Work out the finished part from the listing and answer in its coordinate system (mm). Round coordinates to 2 decimals unless told otherwise and drop trailing zeros. Order: outer loops, then holes, each group sorted by start corner. A loop starts at its lowest first (then second) coordinate and runs counter-clockwise, first axis right, second up. Notation, with made-up numbers: M -29.5,-27 L -21.5,-27 A11 cw -21.5,-23 Z; hole C 8.5,-34.75 d9. An arc over 180 degrees is marked long. Answer as a JSON object with one key per item and string values. Group by question number.
from build123d import *

# Parameters (mm, degrees)
F0_R      = 43.786601
F1_DEPTH  = 63.5
F2_R      = 36.948177
F3_DEPTH  = 127.001
F4_R      = 14.964631
F5_DEPTH  = 177.8
F6_R      = 10.234569
F7_DEPTH  = 177.8
F8_DEPTH  = 127.001
F10_DEPTH = 21.80281
F11_R     = 13.282854
F11_R_2   = 9.414952
F12_DEPTH = 119.06572
F13_R     = 8.242853
F14_DEPTH = 126.54868
F15_R     = 37.892403
F16_DEPTH = 63.501
F17_R     = 10.259839
F18_DEPTH = 185.08291
F19_DEPTH = 161.75664


with BuildPart() as f1:
    # F0 (on Front) → F1 (new body, symmetric)
    with BuildSketch(Plane.XZ):
        Circle(F0_R)
    extrude(amount=F1_DEPTH, both=True)

    # F2 (on face) → F3 (cut, through all)
    with BuildSketch(Plane.XZ.offset(63.5)):
        Circle(F2_R)
    extrude(amount=-F3_DEPTH, mode=Mode.SUBTRACT)

    # F4 (on Right) → F5 (join)
    with BuildSketch(Plane.YZ):
        with Locations((43.817297, 0)):
            Circle(F4_R)
    extrude(amount=F5_DEPTH)

    # F6 (on face) → F7 (cut)
    with BuildSketch(Plane.YZ.offset(177.8)):
        with Locations((43.817297, 0)):
            Circle(F6_R)
    extrude(amount=-F7_DEPTH, mode=Mode.SUBTRACT)

    # F2 (on face) → F8 (cut, through all)
    with BuildSketch(Plane.XZ.offset(63.5)):
        Circle(F2_R)
    extrude(amount=-F8_DEPTH, mode=Mode.SUBTRACT)

    # F9 (on Top) → F10 (join, symmetric)
    with BuildSketch(Plane.XY):
        Polygon((37.235875, -51.78196), (4.975257, -18.238248), (-1.817873, -25.221262), (30.218051, -58.531342), align=None)
    extrude(amount=F10_DEPTH, both=True)

    # F11 (on face) → F12 (join)
    with BuildSketch(Plane(origin=(-13.545415, -13.027284, 0), x_dir=(0.693187, -0.720757, 0), z_dir=(-0.720757, -0.693187, 0))):
        with Locations((40.942468, 0)):
            Circle(F11_R)
        with Locations((40.942468, 0)):
            Circle(F11_R_2, mode=Mode.SUBTRACT)
    extrude(amount=-F12_DEPTH)

    # F13 (on face) → F14 (cut)
    with BuildSketch(Plane(origin=(-13.545415, -13.027284, 0), x_dir=(0.693187, -0.720757, 0), z_dir=(-0.720757, -0.693187, 0))):
        with Locations((42.958759, 0)):
            Circle(F13_R)
    extrude(amount=-F14_DEPTH, mode=Mode.SUBTRACT)

    # F15 (on Front) → F16 (cut, through all)
    with BuildSketch(Plane.XZ):
        Circle(F15_R)
    extrude(amount=F16_DEPTH, mode=Mode.SUBTRACT)

    # F17 (on face) → F18 (cut)
    with BuildSketch(Plane.YZ.offset(177.8)):
        with Locations((43.817297, 0)):
            Circle(F17_R)
    extrude(amount=-F18_DEPTH, mode=Mode.SUBTRACT)

    # F15 (on Front) → F19 (cut)
    with BuildSketch(Plane.XZ):
        Circle(F15_R)
    extrude(amount=-F19_DEPTH, mode=Mode.SUBTRACT)


solid = f1.part
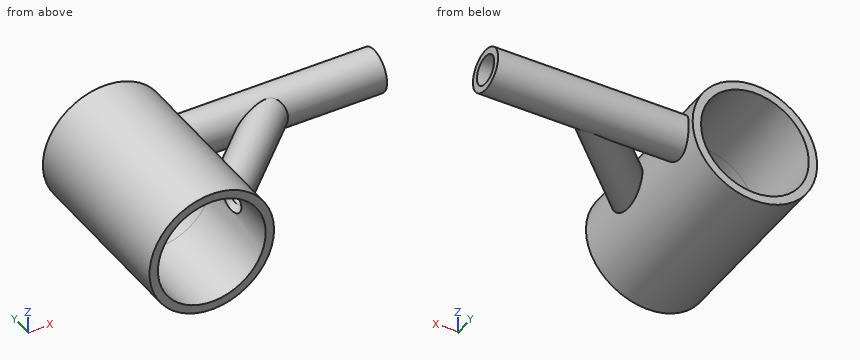
Item 1: Find section C-C (x = 123.5). Give the vertices of the cut face in (y, z), and give its area (3 significant figures).
Item 2: Find section B-B (z = 0). Give the vertices of the cut face in (x, y).
Item 3: Find section D-D (x = 50). Give the number of separate pieces and of enclosed holes in the cut face, and give its area (3 significant figures).
Item 4: Consider L1, parallel to Z at x = 0, y = 27.5; L2, parallel to Y at x = 61, z = 0; L3, parallel to Z at x = 5, y = 55.5. Determine where each line is inside the solid, lowest interval first.
Item 5: Find section A-A (x = 0). Give the vertices of the cut face in (y, z), and give its area (3 significant figures).
Item 6: Each of these flat-tipped pins is pushed along its axis until it touches: pin 1 (4 mm diameter, centred on x = 94.5, z = -11, fed in from +Y); pin 2 (12 mm diameter, centred on y = -37.5, z = -18.5, fed in from +X); pin 3 (3 mm diameter, centred on x = -16.5, y = 28, fed in from +Z); pin 4 (6 mm diameter, centred on x = -12.5, z = -34.5, fed in from +Y). Where does it stop, or does it pass through?
Responses:
{
 "1": {"outline": "C 43.82,0 d29.93; hole C 43.82,0 d20.52", "area": "373 mm^2"},
 "2": {"outline": "M -43.79,-63.5 L -37.89,-63.5 L -37.89,63.5 L -43.79,63.5 Z; M 37.89,-63.5 L 43.79,-63.5 L 43.79,-33.12 L 108.23,28.85 L 177.8,28.85 L 177.8,33.56 L 108.76,33.56 L 37.89,-34.6 Z; M 37.89,-11.72 L 43.79,-6.05 L 43.79,-1.63 L 75.48,28.85 L 80.08,28.85 L 84.97,33.56 L 37.89,33.56 Z; M 37.89,54.08 L 177.8,54.08 L 177.8,58.78 L 43.79,58.78 L 43.79,63.5 L 37.89,63.5 Z; hole M 43.79,3.74 L 69.9,28.85 L 43.79,28.85 Z"},
 "3": {"separate pieces": "2", "enclosed holes": "2", "area": "743 mm^2"},
 "4": {"L1": "z = -43.79 to -37.89, 37.89 to 43.79", "L2": "y = -16.57 to -12.37, 14.92 to 20.29, 28.85 to 33.56, 54.08 to 58.78", "L3": "z = -43.5 to -37.56, 37.56 to 43.5"},
 "5": {"outline": "M -63.5,-43.79 L 63.5,-43.79 L 63.5,-37.89 L -63.5,-37.89 Z; M -63.5,37.89 L 63.5,37.89 L 63.5,43.79 L -63.5,43.79 Z", "area": "1,500 mm^2"},
 "6": {"pin 1": "stops at y = 55.77", "pin 2": "stops at x = 41.96", "pin 3": "stops at z = 41.14", "pin 4": "stops at y = 63.5"}
}
